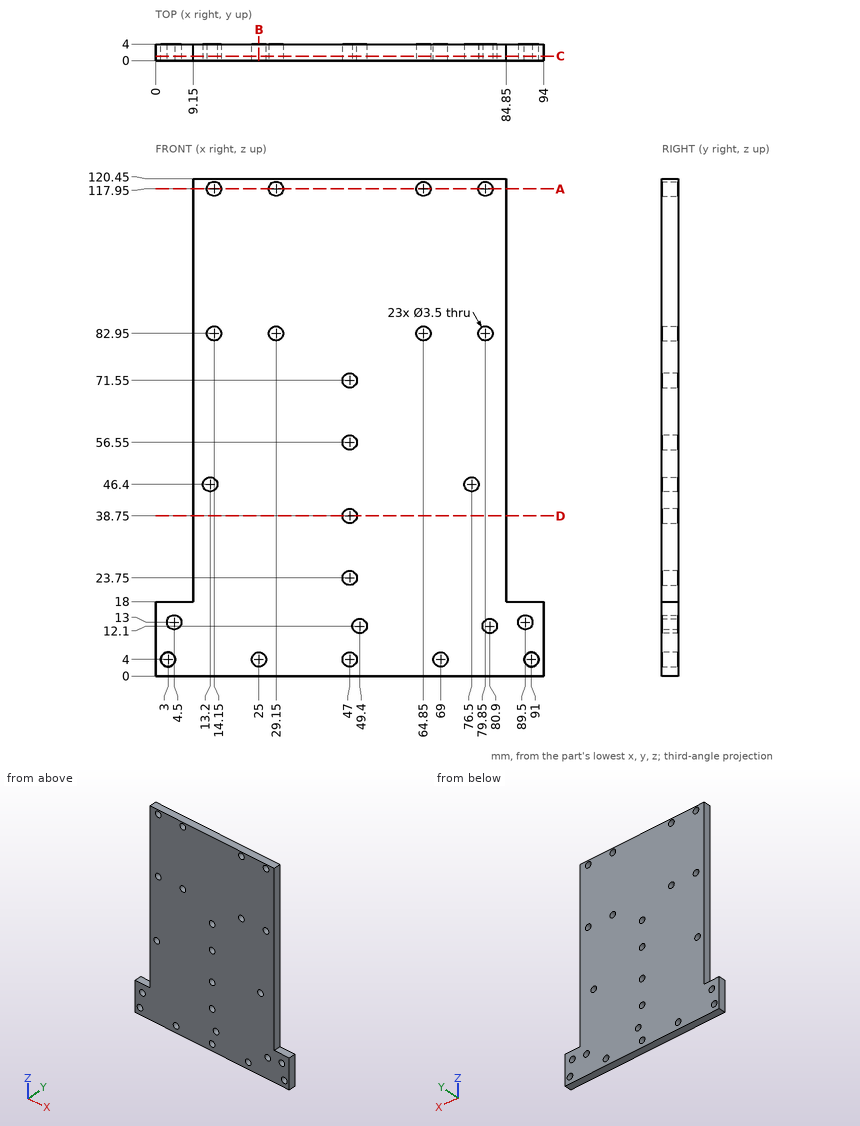
Answer from the drawing. Dimensions are ordinates in mm from the lowest x, y and z of the part. Give positions to 0.01 mm unless a question says otherwise; leave off trailing zeros. Order: outer loops, then holes, each group sorted by start corner. A loop starts at its lowest first (then second) coordinate and runs counter-clockwise, first axis right, second up. Notation, with made-up numbers: (52.5, 27.25) - (60.5, 27.25) arc R19 ccw to (60.5, 44.25) - close; hole circle Ø1 at (-30.75, 46). An arc over 180 degrees is marked (long way). One line per item, written item: value. Start each with the question number.
1. Section D-D, the plane z = 38.75 is taken. Write down the section's boundary in (x, y), then the cut area to 3 significant figures.
2. Each of these flat-tipped pins is pushed along its axis until it touches: pin 1 Ø2 at (x, y) = (90, 2) entering from +Z; pin 2 Ø2 at (x, z) = (29.15, 82.95) entering from +Y; pin 3 Ø1 at (y, z) = (3, 45.5) entering from +X. Where does it stop, or does it pass through?
3. Section A-A, the plane z = 117.95 is taken. Write down the section's boundary in (x, y), then the cut area to 3 significant figures.
4. Section B-B, the plane x = 25 is taken. Write down the section's boundary in (y, z), then the cut area to 3 significant figures.
5. Consider line 1 (X direction, y = 2.3, z = 4); line 2 (X direction, y = 0.25, z = 12); line 3 (X direction, y = 1.1, z = 38.75). Determine where each line is inside the solid, lowest interval first.
6. Section C-C, the plane y = 1.05 is taken. Count the separate pieces of the cut face and the enclosed holes in it, then the cut area to 3 significant figures.
Filled sheet:
1. outline: (9.15, 0) - (45.25, 0) - (45.25, 4) - (9.15, 4) - close; (48.75, 0) - (84.85, 0) - (84.85, 4) - (48.75, 4) - close
1. area: 289 mm²
2. pin 1: z = 18
2. pin 2: through
2. pin 3: x = 84.85
3. outline: (9.15, 0) - (12.4, 0) - (12.4, 4) - (9.15, 4) - close; (15.9, 0) - (27.4, 0) - (27.4, 4) - (15.9, 4) - close; (30.9, 0) - (63.1, 0) - (63.1, 4) - (30.9, 4) - close; (66.6, 0) - (78.1, 0) - (78.1, 4) - (66.6, 4) - close; (81.6, 0) - (84.85, 0) - (84.85, 4) - (81.6, 4) - close
3. area: 247 mm²
4. outline: (0, 0) - (4, 0) - (4, 2.25) - (0, 2.25) - close; (0, 5.75) - (4, 5.75) - (4, 120.45) - (0, 120.45) - close
4. area: 468 mm²
5. line 1: 0 to 1.25, 4.75 to 23.25, 26.75 to 45.25, 48.75 to 67.25, 70.75 to 89.25, 92.75 to 94
5. line 2: 0 to 3.06, 5.94 to 47.65, 51.15 to 79.15, 82.65 to 88.06, 90.94 to 94
5. line 3: 9.15 to 45.25, 48.75 to 84.85
6. separate pieces: 1
6. enclosed holes: 23
6. area: 9,230 mm²
